```python
from build123d import *

# Parameters (mm, degrees)
F0_W      = 126.1496841908
F0_H      = 120.2754974365
F1_DEPTH  = 10.414
F2_W      = 20.2760398388
F2_H      = 22.6492062211
F3_DEPTH  = 122.174
F4_W      = 22.7675586939
F4_H      = 22.8002071381
F5_DEPTH  = 122.174
F6_W      = 23.7396918237
F6_H      = 20.0196914375
F7_DEPTH  = 122.174
F8_W      = 21.2444029748
F8_H      = 21.6576848179
F9_DEPTH  = 122.174
F10_W     = 126.1496841908
F10_H     = 9.857006371
F11_DEPTH = 134.112
F12_W     = 10.8794793487
F12_H     = 112.9197366536
F12_W_2   = 10.2443918586
F12_H_2   = 113.0264736712
F12_W_3   = 10.8346808702
F12_H_3   = 113.1561808288
F12_W_4   = 12.787386775
F12_H_4   = 112.809246406
F13_DEPTH = 25.4


with BuildPart() as f1:
    # F0 (on Top) → F1 (new body)
    with BuildSketch(Plane.XY):
        Rectangle(F0_W, F0_H)
    extrude(amount=F1_DEPTH)

    # F2 (on face) → F3 (join)
    with BuildSketch(Plane(origin=(0, 0, 0), x_dir=(1, 0, 0), z_dir=(0, 0, -1))):
        with Locations((-45.7890219986, 41.4139181376)):
            Rectangle(F2_W, F2_H)
    extrude(amount=F3_DEPTH)

    # F4 (on face) → F5 (join)
    with BuildSketch(Plane(origin=(0, 0, 0), x_dir=(1, 0, 0), z_dir=(0, 0, -1))):
        with Locations((42.81097278, 43.2243607938)):
            Rectangle(F4_W, F4_H)
    extrude(amount=F5_DEPTH)

    # F6 (on face) → F7 (join)
    with BuildSketch(Plane(origin=(0, 0, 0), x_dir=(1, 0, 0), z_dir=(0, 0, -1))):
        with Locations((44.8694061488, -43.2738680393)):
            Rectangle(F6_W, F6_H)
    extrude(amount=F7_DEPTH)

    # F8 (on face) → F9 (join)
    with BuildSketch(Plane(origin=(0, 0, 0), x_dir=(1, 0, 0), z_dir=(0, 0, -1))):
        with Locations((-45.5452147871, -40.8827578649)):
            Rectangle(F8_W, F8_H)
    extrude(amount=F9_DEPTH)

    # F10 (on face) → F11 (join)
    with BuildSketch(Plane.XY.offset(10.414)):
        with Locations((0, -55.2092455328)):
            Rectangle(F10_W, F10_H)
    extrude(amount=F11_DEPTH)

    # F12 (on face) → F13 (cut)
    with BuildSketch(Plane(origin=(0, -50.2807423472, 0), x_dir=(-1, 0, 0), z_dir=(0, 1, 0))):
        with Locations((-43.7446571887, 72.4568422884)):
            Rectangle(F12_W, F12_H)
        with Locations((-13.5027915239, 72.5102107972)):
            Rectangle(F12_W_2, F12_H_2)
        with Locations((13.8100152835, 72.575064376)):
            Rectangle(F12_W_3, F12_H_3)
        with Locations((41.6683144867, 72.4015971646)):
            Rectangle(F12_W_4, F12_H_4)
    extrude(amount=-F13_DEPTH, mode=Mode.SUBTRACT)


solid = f1.part
```
Verification items for the finished model (mm, model axes). A direction names the side the tool comes from. Coordinates: 2 decimals unless noted, no trailing zeros. Order: outer loops, then holes, each group sorted by start corner. A loop starts at its lowest first (then second) coordinate and runs counter-clockwise, first axis right, second up. Notation, with made-up numbers: (60.25, -25) -> (68.25, -25) arc R25 ccw to (68.25, -5) -> close; hole circle Ø5 at (29.5, -18.75). An arc over 180 degrees is marked (long way). Put each result on its own line as item: value. Start each with the question number.
1) Cross-section at B-B (y = -42.5). Enter the section's corners in (x, z), plus the area to 3 significant figures.
2) Material ranges on L1, parallel to Y at x = 50, z = -71; L2, parallel to X at y = 38, z = -20.5; L3, parallel to Z at x = 40.5, y = -13, recorded low to high.
3) Cross-section at D-D (x = -26.5). Enter the section's corners in (y, z), plus the area to 3 significant figures.
4) Cross-section at A-A (z = 80.5). Enter the section's corners in (x, y), plus the area to 3 significant figures.
5) Tool access check on faces 1 (the flat face through (-46, -52.739, -60)), 2 (the flat face through (-35.275, -55, 72)), 3 (the flat face through (43, -54.624, -60)), 4 (the flat face through (-46, 30.054, -60)), 5 (the flat face through (-1, -50.281, 77)). Record the directions out of +Z, -Z, +X, -X, +Y, -Y that give a thin tool (end or side, any length) a straight path to the whole face; none if there is none.
6) Release check for a two-part mould opening along X. For faces 6 (the flat face through (31.427, -43, -60)), 7 (the flat face through (-1, 1, 0)), 8 (the flat face through (56.739, 43, -60)), 9 (the flat face through (45, 33.264, -60)) record: pulls with the +X half, pulls with the -X half, needs draft (parallel to the pull), parting line crosses it, or undercut.
7) Cross-section at C-C (z = -45). Enter the section's corners in (x, y).
8) Go/stop test with flat-tipped pins: pin 1 (17.5 mm diameter, centred on y = 37, z = -78, fed in from -X); pin 2 (5 mm diameter, centred on x = -41.5, y = -55.5, fed in from -Z); pin 3 (12 mm diameter, centred on x = 23, y = 43, fed in from +Z). Record where each tip stops, or that it passes through.
Geometry check:
1. outline: (-63.07, 0) -> (-55.93, 0) -> (-55.93, -122.17) -> (-35.65, -122.17) -> (-35.65, 0) -> (31.43, 0) -> (31.43, -122.17) -> (54.19, -122.17) -> (54.19, 0) -> (63.07, 0) -> (63.07, 10.41) -> (-63.07, 10.41) -> close
1. area: 6,570 mm^2
2. L1: y = -54.62 to -31.82, 33.26 to 53.28
2. L2: x = -56.17 to -34.92, 33 to 56.74
2. L3: z = 0 to 10.41
3. outline: (-60.14, 0) -> (60.14, 0) -> (60.14, 10.41) -> (-50.28, 10.41) -> (-50.28, 144.53) -> (-60.14, 144.53) -> close
3. area: 2,570 mm^2
4. outline: (-63.07, -60.14) -> (-48.06, -60.14) -> (-48.06, -50.28) -> (-63.07, -50.28) -> close; (-35.27, -60.14) -> (-19.23, -60.14) -> (-19.23, -50.28) -> (-35.27, -50.28) -> close; (-8.39, -60.14) -> (8.38, -60.14) -> (8.38, -50.28) -> (-8.39, -50.28) -> close; (18.62, -60.14) -> (38.3, -60.14) -> (38.3, -50.28) -> (18.62, -50.28) -> close; (49.18, -60.14) -> (63.07, -60.14) -> (63.07, -50.28) -> (49.18, -50.28) -> close
4. area: 802 mm^2
5. face 1: -Z, -X, -Y
5. face 2: +Y, -Y
5. face 3: -Z, +X, -X, -Y
5. face 4: -Z, +X, -X
5. face 5: +Z, +X, -X, +Y
6. face 6: undercut
6. face 7: undercut
6. face 8: pulls with the +X half
6. face 9: needs draft
7. outline: (-56.17, 30.05) -> (-34.92, 30.05) -> (-34.92, 51.71) -> (-56.17, 51.71) -> close; (-55.93, -52.74) -> (-35.65, -52.74) -> (-35.65, -30.09) -> (-55.93, -30.09) -> close; (31.43, -54.62) -> (54.19, -54.62) -> (54.19, -31.82) -> (31.43, -31.82) -> close; (33, 33.26) -> (56.74, 33.26) -> (56.74, 53.28) -> (33, 53.28) -> close
8. pin 1: stops at x = -56.17
8. pin 2: stops at z = 0
8. pin 3: stops at z = 10.41
